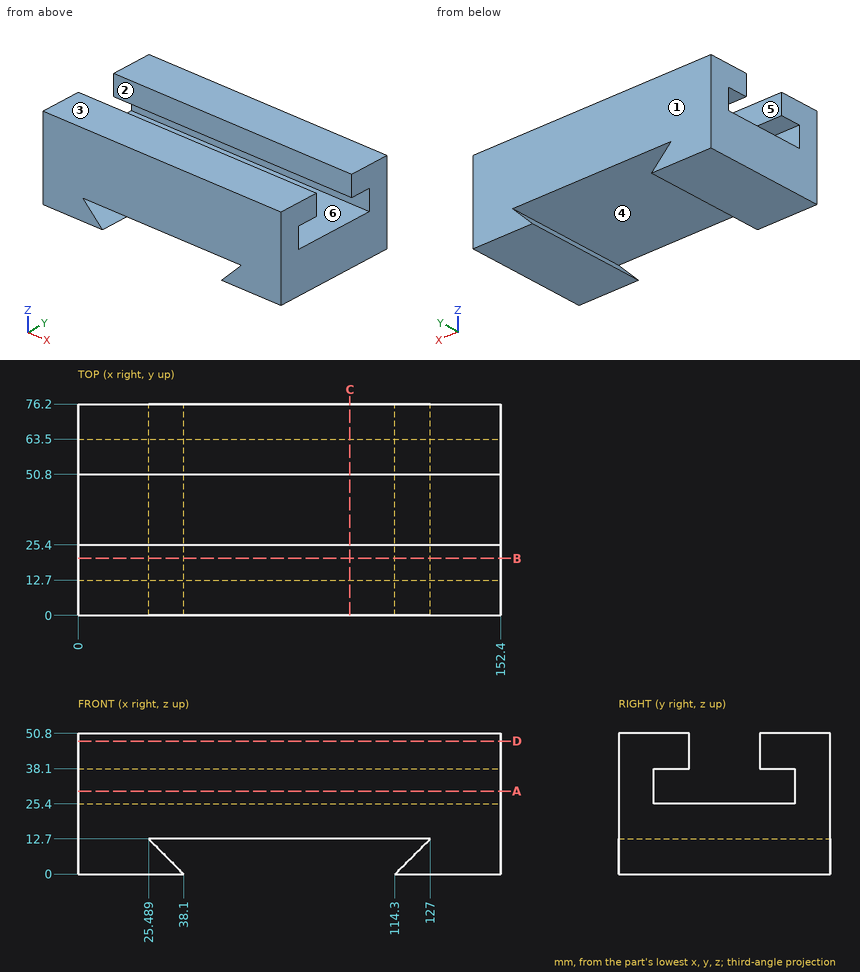
Geometry: see drawing. Coordinates: mm, zero at the bounding-box minimum. A direction names the side the tool comes from. Round coordinates to 2 decimals unless told otherwise and drop trailing zeros. Order: outer loops, then holes, each group sorted by start corner. A loop starts at its lowest first (then second) coordinate and runs counter-clockwise, first axis right, second up. Notation, with made-up numbers: (8.25, 20) - (44.25, 20) arc R30 ccw to (44.25, 42) - close; hole circle Ø5 at (27.25, 58.25). An arc over 180 degrees is marked (long way). One line per question, with ' | ' between items. Start each with the question number.
1) Set-up query: the marked faces 4, 5 and 6. Return all of +Z, -Z, +X, -X, +Y, -Y with unobstructed straight access to the full face (end or side cutting, diameter ignored); none if empty.
2) Cut plane B-B, the plane y = 20.5. Return the cut outline in (x, z), then the cut area to 3 significant figures.
3) Contact query for flat-ended pins moving along their axis: P1, Ø14, axis at x = 99.5, y = 59.5, coming from the -Z side; P2, Ø4, axis at x = 113.5, z = 34, coming from the -Y side. Output: stop coordinate, or through.
4) Cut plane C-C, the plane x = 98. Return the cut outline in (y, z).
5) Pull-direction query (Y, two-part tool) for the marked faces 1, 2 and 3; classes: +Y half, -Y half, draft (parallel to the pull), parting line (faces both ways), or undercut.
6) Ray query, probe 1 along Z at (x, y) = (140, 25); probe 2 along Y at (x, z) = (57.5, 30.5); probe 3 along Z at (x, y) = (52, 52.5). Return the intervals inside material, ascending.
7) Cut plane D-D, the plane z = 48. Return the cut outline in (x, y).
8) Cut plane A-A, the plane z = 30. Return the cut outline in (x, y), then the cut area to 3 significant figures.
Worked out:
1) face 4: +Y, -Y | face 5: +Z, +X, -X | face 6: +X, -X
2) outline: (0, 0) - (38.1, 0) - (25.49, 12.7) - (127, 12.7) - (114.3, 0) - (152.4, 0) - (152.4, 25.4) - (0, 25.4) - close; (0, 38.1) - (152.4, 38.1) - (152.4, 50.8) - (0, 50.8) - close | area: 4,680 mm^2
3) P1: stops at z = 12.7 | P2: stops at y = 0
4) outline: (0, 12.7) - (76.2, 12.7) - (76.2, 50.8) - (50.8, 50.8) - (50.8, 38.1) - (63.5, 38.1) - (63.5, 25.4) - (12.7, 25.4) - (12.7, 38.1) - (25.4, 38.1) - (25.4, 50.8) - (0, 50.8) - close
5) face 1: +Y half | face 2: undercut | face 3: draft
6) probe 1: z = 0 to 25.4, 38.1 to 50.8 | probe 2: y = 0 to 12.7, 63.5 to 76.2 | probe 3: z = 12.7 to 25.4, 38.1 to 50.8
7) outline: (0, 0) - (152.4, 0) - (152.4, 25.4) - (0, 25.4) - close; (0, 50.8) - (152.4, 50.8) - (152.4, 76.2) - (0, 76.2) - close
8) outline: (0, 0) - (152.4, 0) - (152.4, 12.7) - (0, 12.7) - close; (0, 63.5) - (152.4, 63.5) - (152.4, 76.2) - (0, 76.2) - close | area: 3,870 mm^2
